Can you work these out from the drawing? Everything is in mm from the part's minimum corner. A direction names the side the tool comes from. Round coordinates to 2 decimals unless told otherwise and drop trailing zeros. Write each loop counter-clockwise with the first axis right and the second up, starting at its lowest first coordinate (ties: lowest second). Pieces come first, ordered by that corner, then holes. Notation, with made-up numbers: M 48.25,37 L 102.25,37 A7 ccw 102.25,46 Z; hole C 19,-14.75 d10. An arc over 180 degrees is marked long. Use a Markdown table: item, result. Add a question column.
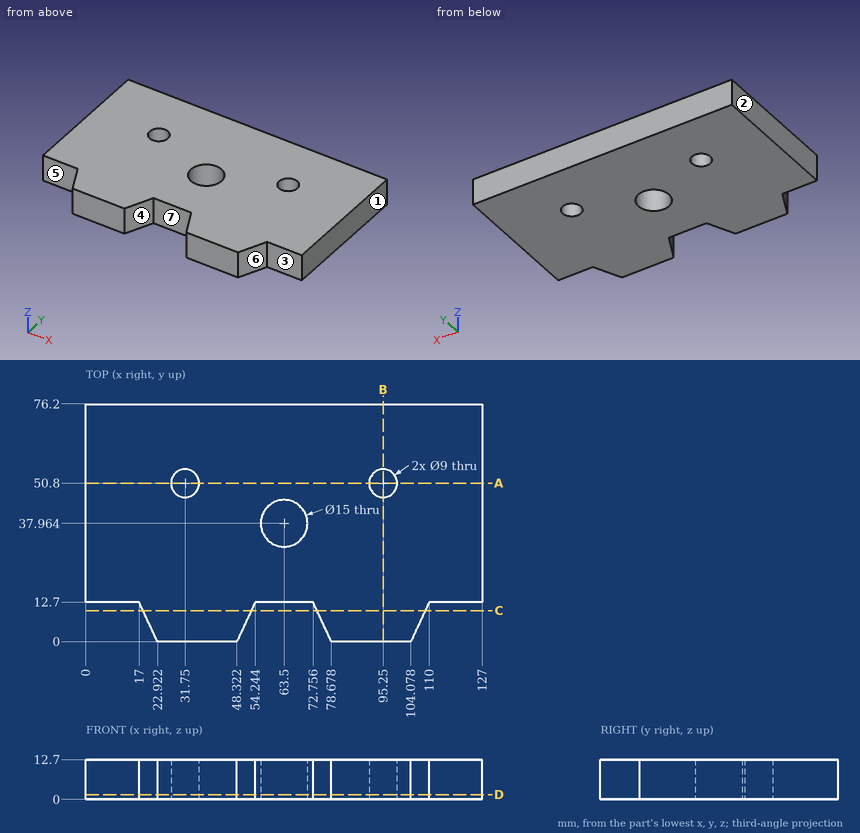
Item 1: For pin 1 Ø3 at (x, z) = (60.5, 4) entering from -Y, with a flat end and sliding along its axis, tell me the tip position at first contact or that it passes through.
Item 2: Imagine slicing it at D-D on z = 1.5. List the corners of the cut face in (x, y) for me, plus the area to 3 significant figures.
Item 3: Imagine slicing it at A-A on y = 50.8. List the corners of the cut face in (x, z) for me, plus the area to 3 significant figures.
Item 4: Imagine slicing it at C-C on y = 10. List the corners of the cut face in (x, z) for me (1 decimal).
Item 5: I need wall thicknesses on probe 1 along Y at (x, z) = (63.5, 6.5); probe 2 along X at (y, z) = (53, 2.25) (1 decimal); probe 3 along Y at (x, z) = (31.75, 5.5). Which ranges of each line are inside material? Lowest first, please. Write a range as from..to.
Item 6: If we mould it in two halves opening along X, with no side actions, what happens to the marked faces 1, 2, 3 and 4? For each: +X half, -X half, draft (parallel to the pull), parting line (faces both ways), or undercut.
Item 7: On a 3-axis mill with a long thin cutter (end or side, diameter ignored), from which of +Z, -Z, +X, -X, +Y, -Y can I reach the whole of each face in a straight line? I mean the marked faces 5, 6 and 7. Say none if no direction works.
Item 8: Imagine slicing it at B-B on x = 95.25. List the corners of the cut face in (y, z) for me.
The answers:
| question | item | result |
|---|---|---|
| 1 | pin 1 | y = 12.7 |
| 2 | outline | M 0,12.7 L 17,12.7 L 22.92,0 L 48.32,0 L 54.24,12.7 L 72.76,12.7 L 78.68,0 L 104.08,0 L 110,12.7 L 127,12.7 L 127,76.2 L 0,76.2 Z; hole C 31.75,50.8 d9; hole C 63.5,37.96 d15; hole C 95.25,50.8 d9 |
| 2 | area | 8,560 mm² |
| 3 | outline | M 0,0 L 27.25,0 L 27.25,12.7 L 0,12.7 Z; M 36.25,0 L 90.75,0 L 90.75,12.7 L 36.25,12.7 Z; M 99.75,0 L 127,0 L 127,12.7 L 99.75,12.7 Z |
| 3 | area | 1,380 mm² |
| 4 | outline | M 18.3,0 L 53,0 L 53,12.7 L 18.3,12.7 Z; M 74,0 L 108.7,0 L 108.7,12.7 L 74,12.7 Z |
| 5 | probe 1 | 12.7..30.46, 45.46..76.2 |
| 5 | probe 2 | 0..27.8, 35.7..91.3, 99.2..127 |
| 5 | probe 3 | 0..46.3, 55.3..76.2 |
| 6 | face 1 | +X half |
| 6 | face 2 | -X half |
| 6 | face 3 | draft |
| 6 | face 4 | undercut |
| 7 | face 5 | +Z, -Z, -X, -Y |
| 7 | face 6 | +Z, -Z, +X, -Y |
| 7 | face 7 | +Z, -Z, -Y |
| 8 | outline | M 0,0 L 46.3,0 L 46.3,12.7 L 0,12.7 Z; M 55.3,0 L 76.2,0 L 76.2,12.7 L 55.3,12.7 Z |
